```python
from build123d import *

# Parameters (mm, degrees)
F0_W      = 25.41
F0_H      = 29.997
F1_DEPTH  = 39.858
F4_D      = 3.3
F4_DEPTH  = 14
F4_TIP    = 0.9914200214
F3_W      = 6.626
F3_H      = 2.444
F5_DEPTH  = 29.998
F6_D      = 12.2
F7_D      = 2.5
F3_R      = 10.961
F8_DEPTH  = 7.15
F9_R      = 7.5
F10_DEPTH = 4.997


with BuildPart() as f1:
    # F0 (on Top) → F1 (new body)
    with BuildSketch(Plane.XY):
        Rectangle(F0_W, F0_H)
    extrude(amount=F1_DEPTH)

    # F4
    with Locations(Plane.XY.offset(39.858)):
        with Locations((-1.25, 4.2395), (-1.25, -4.2395)):
            Hole(F4_D / 2, depth=F4_DEPTH)
            with Locations((0, 0, -(F4_DEPTH + F4_TIP / 2))):  # 118° drill point
                Cone(0, F4_D / 2, F4_TIP, mode=Mode.SUBTRACT)

    # F3 (on face) → F5 (cut, through all)
    with BuildSketch(Plane.XZ.offset(14.9985)):
        with Locations((-1.25, 32.564)):
            Rectangle(F3_W, F3_H)
    extrude(amount=-F5_DEPTH, mode=Mode.SUBTRACT)

    # F6 (through all)
    with Locations(Plane.XZ.offset(14.9985)):
        with Locations((-1.25, 15.589)):
            Hole(F6_D / 2)

    # F7 (through all)
    with Locations(Plane.XZ.offset(14.9985)):
        with Locations((-9.29, 15.589), (6.79, 15.589)):
            Hole(F7_D / 2)

    # F3 (on face) → F8 (cut)
    with BuildSketch(Plane.XZ.offset(14.9985)):
        with Locations((-1.25, 15.589)):
            Circle(F3_R)
    extrude(amount=-F8_DEPTH, mode=Mode.SUBTRACT)

    # F9 (on face) → F10 (cut)
    with BuildSketch(Plane(origin=(0, 14.9985, 0), x_dir=(-1, 0, 0), z_dir=(0, 1, 0))):
        with Locations((1.25, 15.589)):
            Circle(F9_R)
    extrude(amount=-F10_DEPTH, mode=Mode.SUBTRACT)


solid = f1.part
```
Source: CAD feature listing. Evaluate the final solid. Frame: model axes, mm. A direction names the side the tool comes from. Round coordinates to 2 decimals unless told otherwise and drop trailing zeros. Write each loop counter-clockwise with the first axis right and the second up, starting at its lowest first coordinate (ties: lowest second). Pieces come first, ordered by that corner, then holes. Notation, with made-up numbers: M -15.75,33.5 L 15.25,33.5 A17 ccw 15.25,54.5 Z; hole C -10,59 d2. An arc over 180 degrees is marked long. Use CSV: the item, a comma, the result in double quotes. Start each with the question number.
Q1. Access query for faces 5 (the face through (3, -7.848, 11)), 6 (the face through (-1, 0, 33.786)), 7 (the face through (-0.89, 2.63, 36.78)), 8 (the face through (-1.4, 12.535, 23.088)). Directions: +Z, -Z, +X, -X, +Y, -Y. A direction counts if a zero-diameter tool reaches every point of the face in a straight line with its end or side. Return the directions, or none.
Q2. Cut plane D-D on x = 8.5. Output: boundary loops of the cut face in (y, z), plus the area to 3 significant figures.
Q3. Line query: line 1 (Z direction, x = -1.25, y = -10); line 2 (Y direction, x = -1.25, z = 27.1); line 3 (Z direction, x = 6.79, y = 0.5). Output: solid intervals per line, ascending. Write a range as from..to.
Q4. Pull-direction query (Z, two-part tool) for faces 1 (the face through (-2.824, -3.744, 36.779)), 2 (the face through (-1.096, -3.998, 25.039)), 3 (the face through (-1, 0, 31.342)), 4 (the face through (-1.1, 12.53, 8.09)); classes: +Z half, -Z half, draft (parallel to the pull), parting line (faces both ways), or undercut.
Q5. Cut plane B-B on x = -9.29. Output: boundary loops of the cut face in (y, z), plus the area to 3 significant figures.
Q6. Cut plane A-A on y = 12.5. Output: boundary loops of the cut face in (x, z) (3 decimals).
Q7. Cut plane C-C on y = -1. Output: boundary loops of the cut face in (x, z) (3 decimals).
Q8. First-contact query: P1, Ø3, axis at x = -1.25, y = 4.24, coming from the +Z side; P2, Ø5, axis at x = 2, z = 15.5, coming from the +Y side; P3, Ø2.5, axis at x = -1.25, y = 4.24, coming from the +Z side; P4, Ø2, axis at x = -1.25, y = -4.24, coming from the +Z side. Flat tips, straight axial feed; report the tip coordinate or a pass-through.
Results found:
1,face 5,"-Y"
1,face 6,"+Y, -Y"
1,face 7,"+Z"
1,face 8,"+Y"
2,outline,"M -15,0 L 15,0 L 15,39.86 L -15,39.86 L -15,20.6 L -7.85,20.6 L -7.85,10.58 L -15,10.58 Z"
2,area,"1,120 mm^2"
3,line 1,"0..4.63, 26.55..31.34, 33.79..39.86"
3,line 2,"-15..-5.89, -2.59..2.59, 5.89..15"
3,line 3,"0..14.34, 16.84..39.86"
4,face 1,"draft"
4,face 2,"+Z half"
4,face 3,"undercut"
4,face 4,"undercut"
5,outline,"M -15,0 L 15,0 L 15,14.34 L -7.85,14.34 L -7.85,8.14 L -15,8.14 Z; M -15,23.04 L -7.85,23.04 L -7.85,16.84 L 15,16.84 L 15,39.86 L -15,39.86 Z"
5,area,"1,030 mm^2"
6,outline,"M -12.705,0 L 12.705,0 L 12.705,39.858 L -12.705,39.858 Z; hole M -8.671,14.503 A7.5 ccw 6.171,14.503 A1.25 ccw long 6.171,16.675 A7.5 ccw -8.671,16.675 A1.25 ccw long Z; hole M -4.563,31.342 L 2.063,31.342 L 2.063,33.786 L -4.563,33.786 Z"
7,outline,"M -12.705,0 L 12.705,0 L 12.705,39.858 L -12.705,39.858 Z; hole C -9.29,15.589 d2.5; hole C -1.25,15.589 d12.2; hole M -4.563,31.342 L 2.063,31.342 L 2.063,33.786 L -4.563,33.786 Z; hole C 6.79,15.589 d2.5"
8,P1,"z = 25.77"
8,P2,"through"
8,P3,"z = 25.62"
8,P4,"z = 25.47"
